Input: dimensioned drawing with shaded views. Units: mm. Origin: part minimum x, y, z. A direction names the side the tool comes from. Round coordinates to 2 decimals unless told otherwise and drop trailing zeros. Write each loop counter-clockwise with the first axis right and the second up, starting at its lowest first coordinate (ties: lowest second). Pieces come first, ordered by that corner, then holes. Notation, with made-up numbers: M -23,-6.75 L 29,-6.75 A17 cw 29,18.25 Z; hole C 11,68.5 d1. An arc over 180 degrees is marked long. Answer as CSV lines item,"result". Start each with the question number.
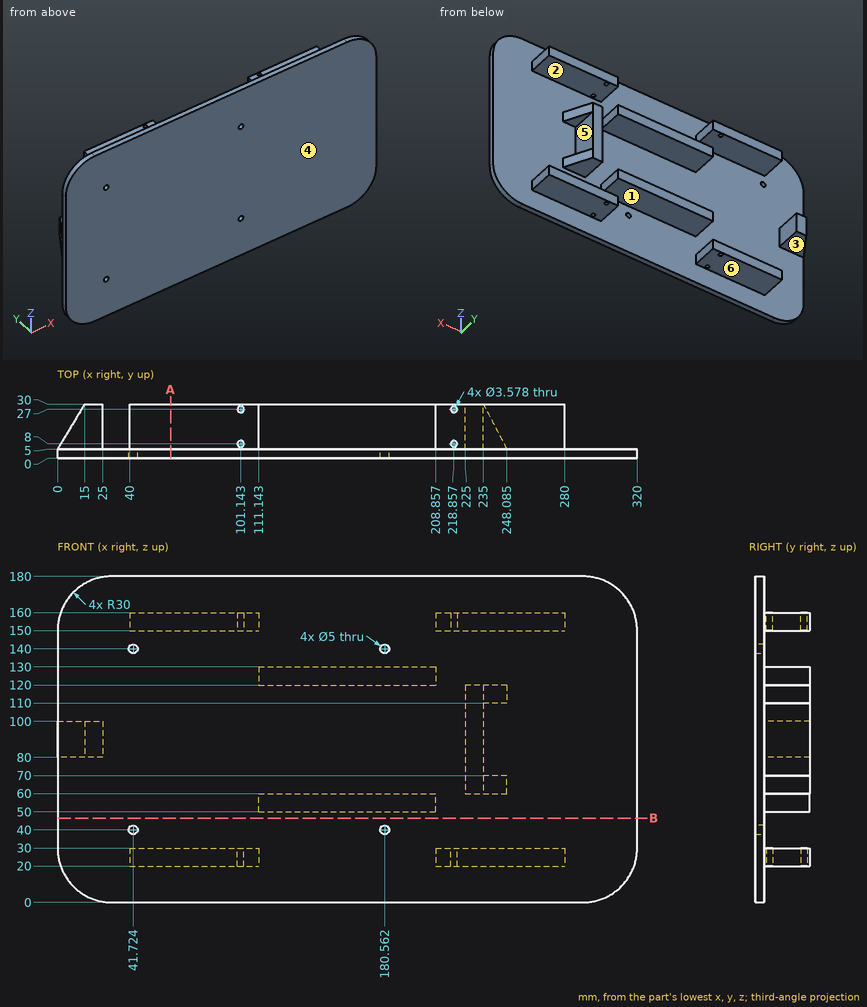
Item 1: Line query: line 1 (X direction, y = 2.75, z = 140); line 2 (Z direction, x = 48, y = 24.5); line 3 (Z direction, x = 120, y = 9.25). Output: solid intervals per line, ascending. Write a range as [from, to].
Item 2: Access query for the marked faces 1, 2 and 3. Directions: +Z, -Z, +X, -X, +Y, -Y. A direction counts if a zero-diameter tool reaches every point of the face in a straight line with its end or side. Return the directions, or none.
Item 3: Cut plane A-A, the plane x = 62.5. Return loops of the section in (y, z), plus the area to 3 significant figures.
Item 4: Draft query along Z for the marked faces 4, 5 and 6. Return one class per face: +Z half, -Z half, draft (parallel to the pull), parting line (faces both ways), or undercut.
Item 5: Cut plane B-B, the plane z = 46.5. Return loops of the section in (x, y).
Item 6: Pin query (flat end, axial travel): pin 1 Ø4 at (x, y) = (239, 26.5) entering from -Z; pin 2 Ø3 at (y, z) = (15.5, 126) entering from +X; pin 3 Ø6 at (x, z) = (174.5, 116) entering from +Y. Return the tip coordinate at first contact, or that it passes through.
Results list:
1,line 1,"[0, 39.22], [44.22, 178.06], [183.06, 320]"
1,line 2,"[20, 30], [150, 160]"
1,line 3,"[50, 60], [120, 130]"
2,face 1,"-Z, +X, -X, +Y"
2,face 2,"+X, -X, +Y"
2,face 3,"-Z, -X, +Y"
3,outline,"M 0,0 L 5,0 L 5,20 L 30,20 L 30,30 L 5,30 L 5,150 L 30,150 L 30,160 L 5,160 L 5,180 L 0,180 Z"
3,area,"1,400 mm²"
4,face 4,"draft"
4,face 5,"undercut"
4,face 6,"-Z half"
5,outline,"M 0,0 L 320,0 L 320,5 L 0,5 Z"
6,pin 1,"z = 20"
6,pin 2,"x = 208.86"
6,pin 3,"y = 5"
